Part model, mm, in its own coordinate system. A direction names the side the tool comes from. Give positions to 0.01 mm unless a question says otherwise; leave off trailing zeros. Write each loop counter-clockwise with the first axis right and the second up, starting at its lowest first coordinate (ties: lowest second). Pieces come first, ordered by that corner, then holes. Notation, with made-up numbers: (6, 35.25) - (15, 35.25) arc R20 ccw to (15, 71.25) - close; hole circle Ø11 at (28.5, -10). An arc over 180 degrees is marked (long way). Answer as a JSON object with one key per item and string values. Group by question number.
```python
from build123d import *

# Parameters (mm, degrees)
F0_W        = 176.9779659808
F0_H        = 50.5181439221
F1_DEPTH    = 50.8
F2_T1_DEPTH = 177.8
F3_W        = 88.7552052736
F3_H        = 41.5458488278
F4_DEPTH    = 5.08


# Not quite as in the source:
# - a fillet or chamfer that OpenCascade refuses, or shapes differently, is made with other operations: its cross-section is extruded or revolved along the edge and cut away or added


with BuildPart() as f1:
    # F0 (on Front) → F1 (new body)
    with BuildSketch(Plane.XZ):
        with Locations((30.3119476885, -8.4089655429)):
            Rectangle(F0_W, F0_H)
    extrude(amount=F1_DEPTH)

    # F2: fillet of radius 25.4 on 4 edges, made by hand

    # F2_s2 → F2_t1 (cut)
    with BuildSketch(Plane.XZ.offset(-63.5)):
        with BuildLine():
            ThreePointArc((-32.7770353019, 16.8501064181), (-50.7375475441, 9.4106186603), (-58.1770353019, -8.5498935819))
            Line((-58.1770353019, -8.5498935819), (-58.1770353019, 16.8501064181))
            Line((-58.1770353019, 16.8501064181), (-32.7770353019, 16.8501064181))
        make_face()
        with BuildLine():
            ThreePointArc((-58.1770353019, -8.268037504), (-50.7375475441, -26.2285497461), (-32.7770353019, -33.668037504))
            Line((-32.7770353019, -33.668037504), (-58.1770353019, -33.668037504))
            Line((-58.1770353019, -33.668037504), (-58.1770353019, -8.268037504))
        make_face()
        with BuildLine():
            ThreePointArc((93.4009306788, 16.8501064181), (111.361442921, 9.4106186603), (118.8009306788, -8.5498935819))
            Line((118.8009306788, -8.5498935819), (118.8009306788, 16.8501064181))
            Line((118.8009306788, 16.8501064181), (93.4009306788, 16.8501064181))
        make_face()
        with BuildLine():
            ThreePointArc((93.4009306788, -33.668037504), (111.361442921, -26.2285497461), (118.8009306788, -8.268037504))
            Line((118.8009306788, -8.268037504), (118.8009306788, -33.668037504))
            Line((118.8009306788, -33.668037504), (93.4009306788, -33.668037504))
        make_face()
    extrude(amount=F2_T1_DEPTH, mode=Mode.SUBTRACT)

    # F3 (on face) → F4 (cut)
    with BuildSketch(Plane.XY.offset(16.8501064181)):
        with Locations((44.3776026368, -25.3384022508)):
            Rectangle(F3_W, F3_H)
    extrude(amount=-F4_DEPTH, mode=Mode.SUBTRACT)


solid = f1.part
```
1) Drill centre lines: line 1 along Z through (x, y) = (39, -19); line 2 along X through (y, z) = (-47.5, 11.5); line 3 along Z through (x, y) = (103, -15.5). Where is each one in solid material? Low to high. Write a range as from..to.
2) Saw through at B-B (y = -9.5). List the corners of the cut face in (x, z), and give its area (3 significant figures).
3) Saw through at C-C (z = -17). List the corners of the cut face in (x, y), and give its area (3 significant figures).
4) Two-plate mould, pull along X, no slides. Class faces 1 (the cylindrical face through (111.11, -25.04, 9.66)), 2 (the flat face through (44, -25, 11.77)), 3 (the cylindrical face through (-50.884, -25.044, -26.081)): +X half, -X half, draft (parallel to the pull), parting line (faces both ways), or undercut.
5) Which spindle directions (+Z, -Z, +X, -X, +Y, -Y) get a long thin tool onto all of the face, cutting with end or side? Do faces 4 (the cylindrical face through (111.113, -25.044, -26.473)), 5 (the flat face through (44, -46.111, 14)). Say none if no direction does.
6) Saw through at A-A (x = 42.5). List the corners of the cut face in (y, z).
7) Drop flat-ended pins along their axis: P1, Ø5.5, axis at y = -15.5, z = 15, coming from the -X side; P2, Ø6, axis at y = -26.5, z = 7, coming from the +X side; P3, Ø2.5, axis at y = -28.5, z = 15, coming from the +X side. Give the stop position or say it passes through.
8) Saw through at D-D (z = 6). List the corners of the cut face in (x, y), and give its area (3 significant figures).
Checks:
{
 "1": {"line 1": "-33.67..11.77", "line 2": "-48.37..108.99", "line 3": "-31.78..14.97"},
 "2": {"outline": "(-58.18, -8.41) arc R25.4 ccw to (-32.78, -33.67) - (93.4, -33.67) arc R25.4 ccw to (118.8, -8.41) arc R25.4 ccw to (93.4, 16.85) - (88.76, 16.85) - (88.76, 11.77) - (0, 11.77) - (0, 16.85) - (-32.78, 16.85) arc R25.4 ccw to start", "area": "7,940 mm2"},
 "3": {"outline": "(-56.63, -50.8) - (117.25, -50.8) - (117.25, 0) - (-56.63, 0) - close", "area": "8,830 mm2"},
 "4": {"face 1": "+X half", "face 2": "undercut", "face 3": "-X half"},
 "5": {"face 4": "-Z, +X, +Y, -Y", "face 5": "+Z"},
 "6": {"outline": "(-50.8, -33.67) - (0, -33.67) - (0, 16.85) - (-4.57, 16.85) - (-4.57, 11.77) - (-46.11, 11.77) - (-46.11, 16.85) - (-50.8, 16.85) - close"},
 "7": {"P1": "x = -47.36", "P2": "x = 115.48", "P3": "x = 105.56"},
 "8": {"outline": "(-53.6, -50.8) - (114.22, -50.8) - (114.22, 0) - (-53.6, 0) - close", "area": "8,530 mm2"}
}
